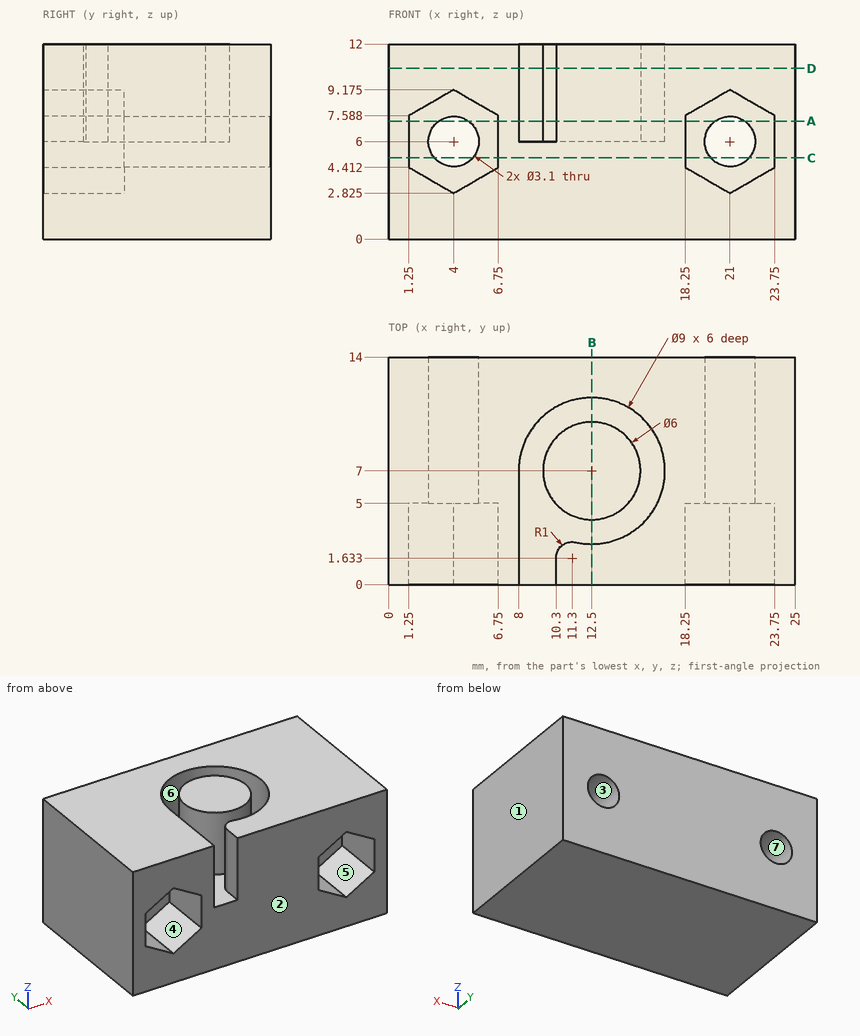
Part print with two shaded views. Sizes in mm from the minimum x, y, z corner. A direction names the side the tool comes from. Round coordinates to 2 decimals unless told otherwise and drop trailing zeros. Write each loop counter-clockwise with the first axis right and the second up, starting at its lowest first coordinate (ties: lowest second). Pieces come first, ordered by that corner, then holes. Notation, with made-up numbers: M -13.5,17.5 L 0.5,17.5 A26 ccw 0.5,44.5 Z; hole C 37,83 d9. An arc over 180 degrees is marked long. Answer as CSV lines item,"result". Start each with the question number.
1) Mould opens along X. For the marked faces 1, 2, 3 and 4 say: +X half, -X half, draft (parallel to the pull), parting line (faces both ways), or undercut.
2) Which spindle directions (+Z, -Z, +X, -X, +Y, -Y) get a long thin tool onto all of the face, cutting with end or side? Do the marked faces 5, 6 and 7. Say none if no direction does.
3) Band-saw the part on A-A (z = 7.25). List the corners of the cut face in (x, y).
4) Drill centre lines: L1, parallel to X at y = 1.25, z = 7; L2, parallel to X at y = 11.75, z = 6.5; L3, parallel to Y at x = 12.25, z = 11.25. Where is each one in solid material? Low to high.
5) Band-saw the part on B-B (x = 12.5). List the corners of the cut face in (y, z).
6) Band-saw the part on D-D (z = 10.5). List the corners of the cut face in (x, y).
7) Band-saw the part on C-C (z = 5). Count the separate pieces of the cut face and the enclosed holes in it, then the cut area to 3 significant figures.
Worked out:
1,face 1,"+X half"
1,face 2,"draft"
1,face 3,"undercut"
1,face 4,"undercut"
2,face 5,"-Y"
2,face 6,"+Z"
2,face 7,"+Y, -Y"
3,outline,"M 0,0 L 1.25,0 L 1.25,5 L 3.08,5 L 3.08,14 L 0,14 Z; M 4.92,5 L 6.75,5 L 6.75,0 L 8,0 L 8,7 A4.5 cw long 11.52,2.61 A1 ccw 10.3,1.63 L 10.3,0 L 18.25,0 L 18.25,5 L 20.08,5 L 20.08,14 L 4.92,14 Z; C 12.5,7 d6; M 21.92,5 L 23.75,5 L 23.75,0 L 25,0 L 25,14 L 21.92,14 Z"
4,L1,"0 to 1.25, 6.75 to 8, 10.3 to 18.25, 23.75 to 25"
4,L2,"0 to 2.53, 5.47 to 19.53, 22.47 to 25"
4,L3,"0 to 2.51, 4.01 to 9.99, 11.49 to 14"
5,outline,"M 0,0 L 14,0 L 14,12 L 11.5,12 L 11.5,6 L 10,6 L 10,12 L 4,12 L 4,6 L 2.5,6 L 2.5,12 L 0,12 Z"
6,outline,"M 0,0 L 8,0 L 8,7 A4.5 cw long 11.52,2.61 A1 ccw 10.3,1.63 L 10.3,0 L 25,0 L 25,14 L 0,14 Z; C 12.5,7 d6"
7,separate pieces,"3"
7,enclosed holes,"0"
7,area,"252 mm²"
